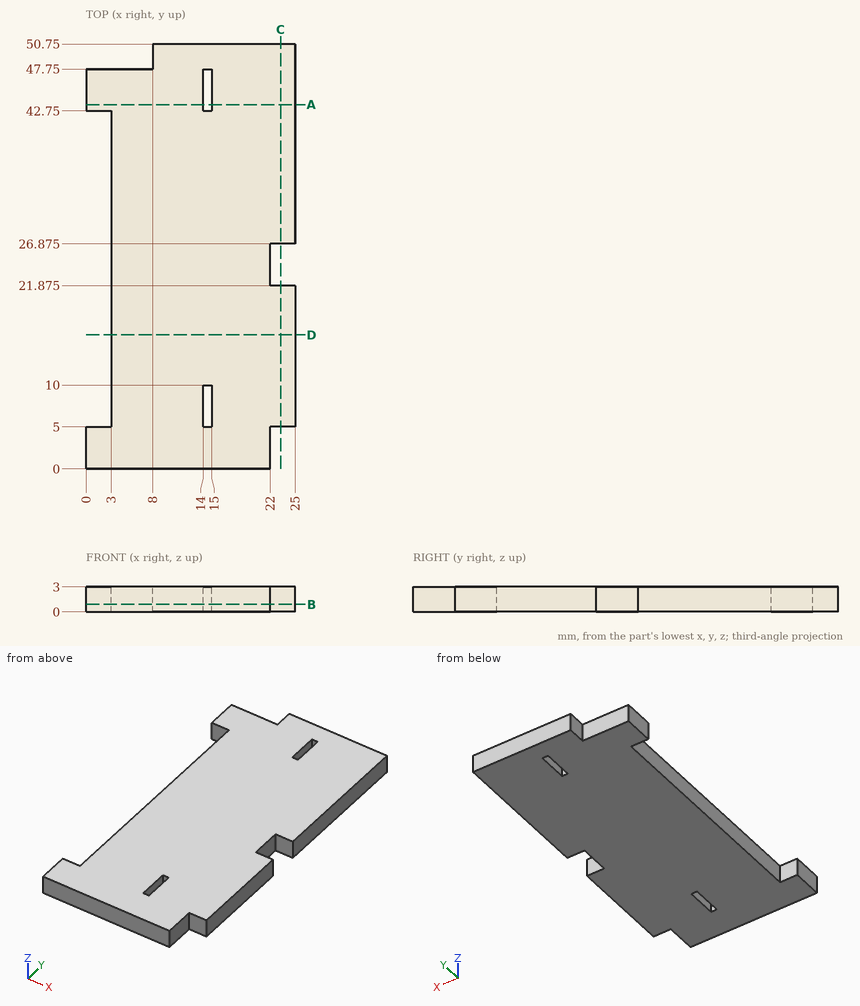
For this review, use the dimensioned drawing (mm, ordinates from the lowest corner) and the shaded views. Round coordinates to 2 decimals unless told otherwise and drop trailing zeros. Write each loop counter-clockwise with the first axis right and the second up, starting at its lowest first coordinate (ties: lowest second). Pieces come first, ordered by that corner, then holes. Notation, with made-up numbers: M 11,65.5 L 55,65.5 A19 cw 55,83.5 Z; hole C 12.5,34.5 d6. An arc over 180 degrees is marked long. Answer as CSV lines item,"result". Start each with the question number.
Q1. Consider section D-D, the plane y = 16. Give the boundary of the cut face in (x, z).
Q2. Consider section B-B, the plane z = 0.9. Give the boundary of the cut face in (x, y) (3 decimals), then the cut area to 3 significant figures.
Q3. Consider section C-C, the plane x = 23.25. Give the boundary of the cut face in (y, z) (3 decimals), then the cut area to 3 significant figures.
Q4. Consider section A-A, the plane y = 43.5. Give the boundary of the cut face in (x, z).
Q5. Clearance check with flat-ended pins moving along their axes: P1, Ø1.5, axis at y = 6.5, z = 1, coming from the -X side; P2, Ø0.9, axis at y = 23.5, z = 1.5, coming from the +X side. State where each tip first meets the part, or that it passes through.
Q6. Wall thickness on line 1 along Y through (x, z) = (23.75, 0.15) (3 decimals); line 2 along Y through (x, z) = (2, 1.75); line 3 along X through (y, z) = (45, 0.2): over which ranges is each line inside the solid? List them lowest first.
Result set:
1,outline,"M 3,0 L 25,0 L 25,3 L 3,3 Z"
2,outline,"M 0,0 L 22,0 L 22,5 L 25,5 L 25,21.875 L 22,21.875 L 22,26.875 L 25,26.875 L 25,50.75 L 8,50.75 L 8,47.75 L 0,47.75 L 0,42.75 L 3,42.75 L 3,5 L 0,5 Z; hole M 14,5 L 15,5 L 15,10 L 14,10 Z; hole M 14,42.75 L 15,42.75 L 15,47.75 L 14,47.75 Z"
2,area,"1,090 mm²"
3,outline,"M 5,0 L 21.875,0 L 21.875,3 L 5,3 Z; M 26.875,0 L 50.75,0 L 50.75,3 L 26.875,3 Z"
3,area,"122 mm²"
4,outline,"M 0,0 L 14,0 L 14,3 L 0,3 Z; M 15,0 L 25,0 L 25,3 L 15,3 Z"
5,P1,"stops at x = 3"
5,P2,"stops at x = 22"
6,line 1,"y = 5 to 21.875, 26.875 to 50.75"
6,line 2,"y = 0 to 5, 42.75 to 47.75"
6,line 3,"x = 0 to 14, 15 to 25"
